from build123d import *

# Parameters (mm, degrees)
SKETCH1_R           = 38.1
SKETCH1_R_2         = 33.0835
BOSS_EXTRUDE1_DEPTH = 6.35
SKETCH2_R           = 38.1
SKETCH2_R_2         = 15.875
BOSS_EXTRUDE2_DEPTH = 3.175


with BuildPart() as part:
    # Sketch1 → Boss-Extrude1 (new body)
    with BuildSketch(Plane(origin=(0, 0, 0), x_dir=(1, 0, 0), z_dir=(0, 1, 0))):
        Circle(SKETCH1_R)
        Circle(SKETCH1_R_2, mode=Mode.SUBTRACT)
    extrude(amount=-BOSS_EXTRUDE1_DEPTH)

    # Sketch2 → Boss-Extrude2 (add)
    with BuildSketch(Plane(origin=(0, 0, 0), x_dir=(1, 0, 0), z_dir=(0, 1, 0))):
        Circle(SKETCH2_R)
        Circle(SKETCH2_R_2, mode=Mode.SUBTRACT)
    extrude(amount=BOSS_EXTRUDE2_DEPTH)


solid = part.part
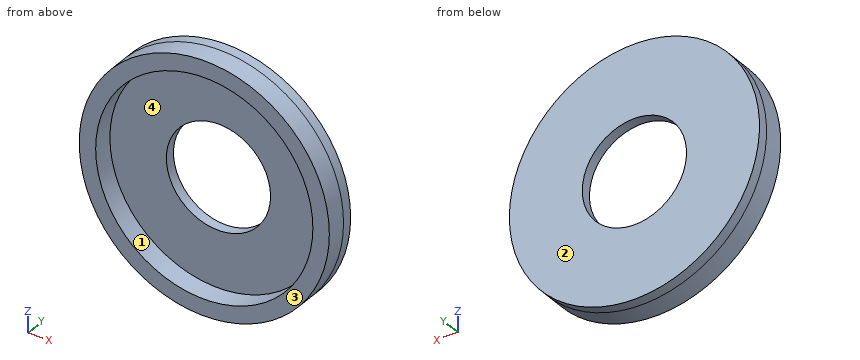
Can you work these out from the model? Positions are in its coordinate system, mm. Face numbers are marked on the shaded views. A direction names the side the tool comes from. Coordinates: 2 decimals unless noted, no trailing zeros. Loops run counter-clockwise (first coordinate to the right, second up) from the corner with the lowest first, then second, coordinate; pieces in that order, holes last. Notation, with made-up numbers: (81.5, -17.5) - (117.5, -17.5) arc R36 ccw to (117.5, 20.5) - close; hole circle Ø3 at (40.25, 45). An arc over 180 degrees is marked (long way). Put each result on its own line as item: value. Start each with the question number.
Item 1: If we mould it in two halves opening along Z, with no side actions, what happens to the marked faces 3 and 4? For each: +Z half, -Z half, draft (parallel to the pull), parting line (faces both ways), or undercut.
Item 2: Suppose I cut it at D-D (x = 24.5). Please give me the cut outline in (y, z) (3 decimals), and give its area (3 significant figures).
Item 3: Which directions (+Z, -Z, +X, -X, +Y, -Y) give clear straight access to the entire face, cutting with the end or side of a thin tool? Please do the marked faces 1 and 2.
Item 4: If I drill on line 1 along X through (y, z) = (1.25, 0) (3 decimals); line 2 along Z through (x, y) = (0, -1.5), over which ranges is the centre line in solid material (lowest first)?
Item 5: Suppose I cut it at C-C (y = -3.75). Please give me the cut outline in (x, z), and give its area (3 significant figures).
Item 6: For pin 1 (2 mm diameter, centred on x = 14.5, y = -4.5, fed in from +Z); pin 2 (1 mm diameter, centred on y = -3, z = 1.5, fed in from -X); pin 3 (10 mm diameter, centred on x = -11.5, z = 11.5, fed in from -Y), each with a flat end and sliding along its axis, tell me the tip position at first contact or that it passes through.
Here are the results:
1. face 3: draft
1. face 4: undercut
2. outline: (-6.35, -29.178) - (3.175, -29.178) - (3.175, 29.178) - (-6.35, 29.178) - (-6.35, 22.232) - (0, 22.232) - (0, -22.232) - (-6.35, -22.232) - close
2. area: 273 mm²
3. face 1: -Y
3. face 2: +Z, -Z, +X, -X, +Y
4. line 1: -38.1 to -15.875, 15.875 to 38.1
4. line 2: -38.1 to -33.08, 33.08 to 38.1
5. outline: circle Ø76.2 at (0, 0); hole circle Ø66.17 at (0, 0)
5. area: 1,120 mm²
6. pin 1: z = 35.63
6. pin 2: x = -38.09
6. pin 3: y = 0
